from build123d import *

# Parameters (mm, degrees)
F3_R            = 1
F4_R            = 3.5
F5_DEPTH        = 30.001
F5_COPIES_COUNT = 3
F7_DEPTH        = 25


# Not quite as in the source:
# - a fillet or chamfer that OpenCascade refuses, or shapes differently, is made with other operations: its cross-section is extruded or revolved along the edge and cut away or added
# - a pattern or mirror of a feature is missing from the dataset's text; its kind, count and spacing are read off the source's solid


with BuildPart() as f1:
    # F0 (on Front) → F1 (revolve)
    with BuildSketch(Plane.XZ):
        with BuildLine():
            Line((30, 50), (0, 50))
            Line((0, 50), (0, 37))
            ThreePointArc((0, 37), (15.5080624193, 34.1576191054), (29, 26))
            Line((29, 26), (30, 26))
            Line((30, 26), (30, 50))
        make_face()
    revolve(axis=Axis((-20.2939212322, 0, 0), (-1, 0, 0)))

    # F2: fillet of radius 2 on 1 edges, made by hand

    # F2_s1 → F2_t2 (revolve, cut)
    with BuildSketch(Plane.XZ):
        with BuildLine():
            ThreePointArc((29.7489495613, 26), (29.0553262341, 26.1241304203), (28.447802662, 26.4811133201))
            ThreePointArc((28.447802662, 26.4811133201), (28.7249086192, 26.241712774), (29, 26))
            Line((29, 26), (29.7489495613, 26))
        make_face()
    revolve(axis=Axis((29, 0, 0), (-1, 0, 0)), mode=Mode.SUBTRACT)

    # F3
    f3_edges = [f1.edges().sort_by_distance(p)[0] for p in [
        (0, 0, -37),
    ]]
    fillet(f3_edges, radius=F3_R)

    # F4 (on face) → F5 (cut, through all)
    with BuildSketch(Plane(origin=(0, 0, 0), x_dir=(0, -1, 0), z_dir=(-1, 0, 0))):
        with Locations((43, 0)):
            Circle(F4_R)
    f5 = extrude(amount=-F5_DEPTH, mode=Mode.SUBTRACT)

    # F5_copies: F5 ×3 about axis
    f5_copies_axis = Axis((0, 0, 0), (1, 0, 0))
    for i in range(1, F5_COPIES_COUNT):
        add(f5.rotate(f5_copies_axis, i * 360 / F5_COPIES_COUNT), mode=Mode.SUBTRACT)

    # F6 (on face) → F7 (cut)
    with BuildSketch(Plane.YZ.offset(30)):
        with BuildLine():
            ThreePointArc((44.0317802314, 23.6897093619), (43.3012701892, 25), (42.5317802314, 26.2877855733))
            Line((42.5317802314, 26.2877855733), (21.7291570127, 14.2773854581))
            ThreePointArc((21.7291570127, 14.2773854581), (22.5166604984, 13), (23.2291570127, 11.6793092467))
            Line((23.2291570127, 11.6793092467), (44.0317802314, 23.6897093619))
        make_face()
        with BuildLine():
            Line((-23.2291570127, -11.6793092467), (-44.0317802314, -23.6897093619))
            ThreePointArc((-44.0317802314, -23.6897093619), (-43.3012701892, -25), (-42.5317802314, -26.2877855733))
            Line((-42.5317802314, -26.2877855733), (-21.7291570127, -14.2773854581))
            ThreePointArc((-21.7291570127, -14.2773854581), (-22.5166604984, -13), (-23.2291570127, -11.6793092467))
        make_face()
    extrude(amount=-F7_DEPTH, mode=Mode.SUBTRACT)


solid = f1.part
Input: part model. Units: mm. Frame: model coordinates. A direction names the side the tool comes from. Round coordinates to 2 decimals unless told otherwise and drop trailing zeros. Order: outer loops, then holes, each group sorted by start corner. A loop starts at its lowest first (then second) coordinate and runs counter-clockwise, first axis right, second up. Notation, with made-up numbers: (82.25, 16.25) - (118.25, 16.25) arc R23 ccw to (118.25, 54.25) - close; hole circle Ø4 at (73.5, 51). An arc over 180 degrees is marked (long way). Use a Markdown table: item, result.
1. First-contact query: pin 1 (1 mm diameter, centred on x = 19, z = -8, fed in from -Y); pin 2 (6 mm diameter, centred on x = 22, y = -30, fed in from -Z); pin 3 (1.5 mm diameter, centred on x = 13.5, z = 29.5, fed in from -Y). Flat tips, straight axial feed; report the tip coordinate or a pass-through.
Evaluation:
| item | result |
|---|---|
| pin 1 | y = -49.43 |
| pin 2 | z = -42.08 |
| pin 3 | y = -40.91 |
2. Section D-D on z = -43.5. Return the cut outline in (x, y), then the cut area to 3 significant figures.
Evaluation:
| item | result |
|---|---|
| outline | (0, -24.65) - (30, -24.65) - (30, 24.65) - (0, 24.65) - close |
| area | 1,480 mm^2 |
3. Access query for faces 1 (the face through (5, 37, 21)), 2 (the face through (14.79, -39.503, 0.154)). Directions: +Z, -Z, +X, -X, +Y, -Y. A direction counts if a zero-diameter tool reaches every point of the face in a straight line with its end or side. Return the directions, or none.
Evaluation:
| item | result |
|---|---|
| face 1 | +X |
| face 2 | +X, -X |
4. Material intervals for probe 1 along Y at (x, z) = (25, 19.5) (3 decimals); probe 2 along Y at (x, z) = (26.5, 20); probe 3 along Z at (x, y) = (15, 21.5), sorted ascending.
Evaluation:
| item | result |
|---|---|
| probe 1 | -46.041 to -21.665, 21.665 to 30.775, 36.775 to 46.041 |
| probe 2 | -45.83 to -19.67, 19.67 to 31.64, 37.64 to 45.83 |
| probe 3 | -45.14 to -40.74, -33.74 to -26.79, 26.79 to 33.74, 40.74 to 45.14 |
5. Section A-A on z = 0. State how many separate pieces and enclosed holes the cut face has, then the cut area to 3 significant figures.
Evaluation:
| item | result |
|---|---|
| separate pieces | 3 |
| enclosed holes | 0 |
| area | 792 mm^2 |
6. Mould query, pull axis Y, two halves, no side actions, for faces 3 (the face through (20.453, -35.796, -18.935)), 4 (the face through (0, 34, 18)), 5 (the face through (14.79, 15.02, 47.69)). Classes: +Y half, -Y half, draft (parallel to the pull), parting line (faces both ways), or undercut.
Evaluation:
| item | result |
|---|---|
| face 3 | undercut |
| face 4 | draft |
| face 5 | parting line |
